from build123d import *

# Parameters (mm, degrees)
SKETCH_1_R          = 3
EXTRUDE_1_DEPTH     = 30
SKETCH_2_R          = 1
CUT_EXTRUDE_1_DEPTH = 30
SKETCH_3_R          = 2
CUT_EXTRUDE_2_DEPTH = 20
CHAMFER_1_SIZE      = 1
CHAMFER_2_SIZE      = 0.2


with BuildPart() as part:
    # Эскиз1 → Бобышка-Вытянуть1 (new body)
    with BuildSketch(Plane.XY):
        Circle(SKETCH_1_R)
    extrude(amount=EXTRUDE_1_DEPTH)

    # Эскиз2 → Вырез-Вытянуть1 (cut)
    with BuildSketch(Plane.XY.offset(30)):
        Circle(SKETCH_2_R)
    extrude(amount=-CUT_EXTRUDE_1_DEPTH, mode=Mode.SUBTRACT)

    # Эскиз3 → Вырез-Вытянуть2 (cut)
    with BuildSketch(Plane.XY.offset(30)):
        Circle(SKETCH_3_R)
    extrude(amount=-CUT_EXTRUDE_2_DEPTH, mode=Mode.SUBTRACT)

    # Фаска1
    chamfer_1_edges = [part.edges().sort_by_distance(p)[0] for p in [
        (-1, 0, 0),
    ]]
    chamfer(chamfer_1_edges, length=CHAMFER_1_SIZE)

    # Фаска2
    chamfer_2_edges = [part.edges().sort_by_distance(p)[0] for p in [
        (-3, 0, 0),
        (-3, 0, 30),
    ]]
    chamfer(chamfer_2_edges, length=CHAMFER_2_SIZE)


solid = part.part
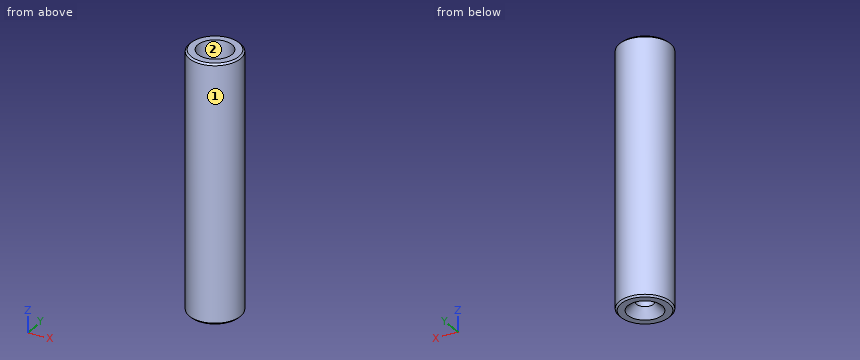
Verification items for the finished model (mm, model axes). Face numbers are marked on the shaded views. Coordinates: 2 decimals unless noted, no trailing zeros. Order: outer loops, then holes, each group sorted by start corner. A loop starts at its lowest first (then second) coordinate and runs counter-clockwise, first axis right, second up. Notation, with made-up numbers: M 78,-37.75 L 125,-37.75 A38 cw 125,1.25 Z; hole C -34.75,-15 d6. An arc over 180 degrees is marked long. Return JSON: item names as keys, results as strings.
1) Cross-section at D-D, the plane z = 9.75. Record the boundary of the cut face in (x, y), and give its area (3 significant figures).
Answer list:
{"outline": "C 0,0 d6; hole C 0,0 d2", "area": "25.1 mm2"}
2) Cross-section at C-C, the plane z = 25.5. Record the boundary of the cut face in (x, y).
Answer list:
{"outline": "C 0,0 d6; hole C 0,0 d4"}
3) Cross-section at A-A, the plane x = 0. Record the boundary of the cut face in (y, z), and give its area (3 significant figures).
Answer list:
{"outline": "M -3,0.2 L -2.8,0 L -2,0 L -1,1 L -1,10 L -2,10 L -2,30 L -2.8,30 L -3,29.8 Z; M 1,1 L 2,0 L 2.8,0 L 3,0.2 L 3,29.8 L 2.8,30 L 2,30 L 2,10 L 1,10 Z", "area": "78.9 mm2"}
4) Thickness scan on L1, parallel to Y at x = 0, z = 17.5; L2, parallel to Y at x = 0, z = 3; L3, parallel to X at y = -0.9, z = 11.5. Record the ranges inside material, lowest first. Write a range as [from, to].
Answer list:
{"L1": "[-3, -2], [2, 3]", "L2": "[-3, -1], [1, 3]", "L3": "[-2.86, -1.79], [1.79, 2.86]"}
5) Gauge pin test, flat end, axial feed: pin 1 (2.5 mm diameter, centred on x = 0, y = 0, fed in from +Z). Record the tip position at first contact, or that the pin passes through.
Answer list:
{"pin 1": "z = 10"}
6) Release check for a two-part mould opening along Y. For the marked faces 1 and 2 record: +Y half, -Y half, draft (parallel to the pull), parting line (faces both ways), or undercut.
Answer list:
{"face 1": "parting line", "face 2": "undercut"}
